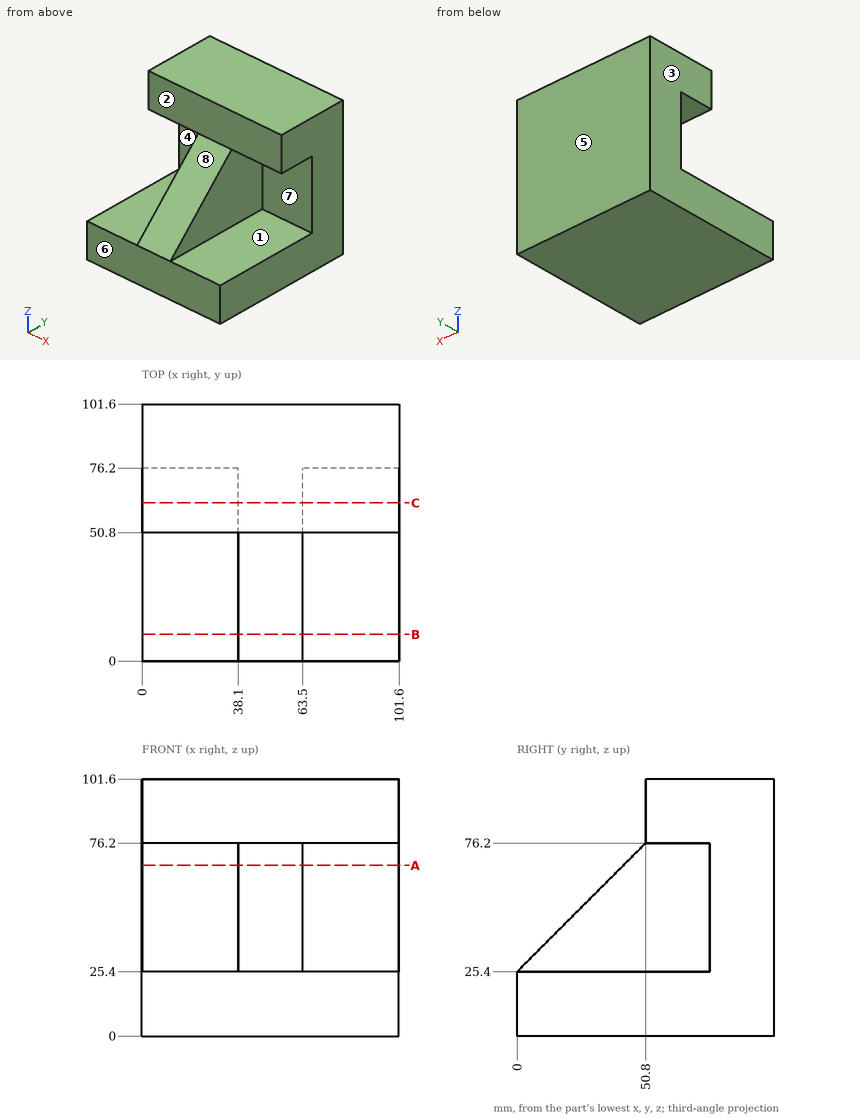
Design review of the part shown in the three views and the two pictorial views. Dimensions are in mm from the part's minimum x, y and z. A direction names the side the tool comes from. Coordinates: 2 decimals unless noted, no trailing zeros. Order: outer loops, then holes, each group sorted by start corner. A loop starts at its lowest first (then second) coordinate and runs counter-clockwise, first axis right, second up. Notation, with made-up numbers: (28.5, 13.5) -> (62.5, 13.5) arc R11 ccw to (62.5, 24.5) -> close; hole circle Ø9 at (-32.75, 24). An arc over 180 degrees is marked (long way). Use one line per item in the form item = value. Start each with the question number.
(1) Add section B-B on y = 10.5. State the section outline as (x, z) points, plus the area to 3 significant figures.
(2) Add section C-C on y = 62.5. State the section outline as (x, z) points, plus the area to 3 significant figures.
(3) For the marked faces 1, 2, 3, 4 and 5, list the 3-axis set-ups (+Z, -Z, +X, -X, +Y, -Y) from which the entire face can be reached by the end or side of a thin tool; tool diameter is ignored.
(4) The part is to be moulded in two halves that separate along Z. For the marked faces 6, 7 and 8, say which applies: +Z half, -Z half, draft (parallel to the pull), parting line (faces both ways), or undercut.
(5) Insertion check: pin 1 (19 mm diameter, centred on x = 10, z = 51, fed in from -Y); pin 2 (12 mm diameter, centred on y = 64, z = 53.5, fed in from +X); pin 3 (10 mm diameter, centred on x = 73.5, z = 83, fed in from -Y). Each pin has a flat end and moves straight along its axis. Give the tip position at first contact, or say it passes through.
(6) Add section A-A on z = 67.5. State the section outline as (x, y) points.
(7) For probe 1 along Z at (x, y) = (76, 57); probe 2 along Y at (x, z) = (16.5, 29); probe 3 along Z at (x, y) = (71, 18.5), list the stretches that pass through material, from the lowest coordinate up.
Answer block:
q1.outline = (0, 0) -> (101.6, 0) -> (101.6, 25.4) -> (63.5, 25.4) -> (63.5, 35.9) -> (38.1, 35.9) -> (38.1, 25.4) -> (0, 25.4) -> close
q1.area = 2,850 mm²
q2.outline = (0, 0) -> (101.6, 0) -> (101.6, 25.4) -> (63.5, 25.4) -> (63.5, 76.2) -> (101.6, 76.2) -> (101.6, 101.6) -> (0, 101.6) -> (0, 76.2) -> (38.1, 76.2) -> (38.1, 25.4) -> (0, 25.4) -> close
q2.area = 6,450 mm²
q3.face_1 = +X, -Y
q3.face_2 = +Z, +X, -X, -Y
q3.face_3 = +Z, -Z, -X, +Y, -Y
q3.face_4 = -X, -Y
q3.face_5 = +Z, -Z, +X, -X, +Y
q4.face_6 = draft
q4.face_7 = undercut
q4.face_8 = +Z half
q5.pin_1 = 76.2
q5.pin_2 = 63.5
q5.pin_3 = 50.8
q6.outline = (0, 76.2) -> (38.1, 76.2) -> (38.1, 42.1) -> (63.5, 42.1) -> (63.5, 76.2) -> (101.6, 76.2) -> (101.6, 101.6) -> (0, 101.6) -> close
q7.probe_1 = 0 to 25.4, 76.2 to 101.6
q7.probe_2 = 76.2 to 101.6
q7.probe_3 = 0 to 25.4
